from build123d import *

# Parameters (mm, degrees)
BOSS_EXTRUDE1_DEPTH     = 16.316743
CUT_EXTRUDE1_DEPTH      = 16.04
CUT_EXTRUDE1_DEPTH_BACK = 16.96
CUT_EXTRUDE2_DEPTH      = 29
CUT_EXTRUDE2_DEPTH_BACK = 29


with BuildPart() as part:
    # Sketch3 → Boss-Extrude1 (new body)
    with BuildSketch(Plane(origin=(0, 0, 0), x_dir=(1, 0, 0), z_dir=(0, 1, 0))):
        Polygon((-28, 15.96), (28, 15.96), (28, -15.04), (12.57, -15.04), (8.79, -11.59), (8.79, -11.02), (12.24, -7.24), (12.24, 0), (-12.24, 0), (-12.24, -7.24), (-8.79, -11.02), (-8.79, -11.59), (-12.57, -15.04), (-28, -15.04), align=None)
    extrude(amount=-BOSS_EXTRUDE1_DEPTH)

    # Sketch4 → Cut-Extrude1 (cut, two sides)
    with BuildSketch(Plane.XY) as cut_extrude1_sk:
        Polygon((28, -3.175), (28, -4.282415891), (20.400144244, -3.728707945), align=None)
        Polygon((28, -4.282415891), (28, -5.389831781), (20.400144244, -4.836123836), align=None)
        Polygon((28, -5.389831781), (28, -6.497247672), (20.400144244, -5.943539726), align=None)
        Polygon((28, -6.497247672), (28, -7.604663562), (20.400144244, -7.050955617), align=None)
        Polygon((28, -7.604663562), (28, -8.712079453), (20.400144244, -8.158371507), align=None)
        Polygon((28, -8.712079453), (28, -9.819495343), (20.400144244, -9.265787398), align=None)
        Polygon((20.400144244, -10.373203288), (28, -10.926911234), (28, -9.819495343), align=None)
        Polygon((28, -10.926911234), (28, -12.034327124), (20.400144244, -11.480619179), align=None)
        Polygon((28, -12.034327124), (28, -13.141743015), (20.400144244, -12.588035069), align=None)
        Polygon((-28, -13.141743015), (-28, -12.034327124), (-20.400144244, -12.588035069), align=None)
        Polygon((-28, -10.926911234), (-20.400144244, -11.480619179), (-28, -12.034327124), align=None)
        Polygon((-28, -10.926911234), (-28, -9.819495343), (-20.400144244, -10.373203288), align=None)
        Polygon((-28, -8.712079453), (-20.400144244, -9.265787398), (-28, -9.819495343), align=None)
        Polygon((-28, -7.604663562), (-20.400144244, -8.158371507), (-28, -8.712079453), align=None)
        Polygon((-28, -6.497247672), (-20.400144244, -7.050955617), (-28, -7.604663562), align=None)
        Polygon((-28, -5.389831781), (-20.400144244, -5.943539726), (-28, -6.497247672), align=None)
        Polygon((-28, -4.282415891), (-20.400144244, -4.836123836), (-28, -5.389831781), align=None)
        Polygon((-28, -3.175), (-20.400144244, -3.728707945), (-28, -4.282415891), align=None)
    extrude(amount=CUT_EXTRUDE1_DEPTH, mode=Mode.SUBTRACT)
    extrude(cut_extrude1_sk.sketch, amount=-CUT_EXTRUDE1_DEPTH_BACK, mode=Mode.SUBTRACT)

    # Sketch5 → Cut-Extrude2 (cut, two sides)
    with BuildSketch(Plane(origin=(0, 0, 0), x_dir=(0, 0, -1), z_dir=(1, 0, 0))) as cut_extrude2_sk:
        Polygon((15.96, -3.175), (15.96, -4.282415891), (8.360144244, -3.728707945), align=None)
        Polygon((8.360144244, -4.836123836), (15.96, -5.389831781), (15.96, -4.282415891), align=None)
        Polygon((15.96, -5.389831781), (15.96, -6.497247672), (8.360144244, -5.943539726), align=None)
        Polygon((8.360144244, -7.050955617), (15.96, -7.604663562), (15.96, -6.497247672), align=None)
        Polygon((15.96, -7.604663562), (15.96, -8.712079453), (8.360144244, -8.158371507), align=None)
        Polygon((8.360144244, -9.265787398), (15.96, -9.819495343), (15.96, -8.712079453), align=None)
        Polygon((15.96, -9.819495343), (15.96, -10.926911234), (8.360144244, -10.373203288), align=None)
        Polygon((8.360144244, -11.480619179), (15.96, -12.034327124), (15.96, -10.926911234), align=None)
        Polygon((15.96, -12.034327124), (15.96, -13.141743015), (8.360144244, -12.588035069), align=None)
    extrude(amount=CUT_EXTRUDE2_DEPTH, mode=Mode.SUBTRACT)
    extrude(cut_extrude2_sk.sketch, amount=-CUT_EXTRUDE2_DEPTH_BACK, mode=Mode.SUBTRACT)


solid = part.part
Part model, mm, in its own coordinate system. Give positions to 0.01 mm unless a question says otherwise; leave off trailing zeros. Loops run counter-clockwise (first coordinate to the right, second up) from the corner with the lowest first, then second, coordinate; pieces in that order, holes last.
(1) Band-saw the part on D-D (x = 17.5). Write the cut outline in (y, z) (1 decimal).
Return value:
outline: (-16.3, -16) - (-13.1, -16) - (-12.6, -8.4) - (-12, -16) - (-11.5, -8.4) - (-10.9, -16) - (-10.4, -8.4) - (-9.8, -16) - (-9.3, -8.4) - (-8.7, -16) - (-8.2, -8.4) - (-7.6, -16) - (-7.1, -8.4) - (-6.5, -16) - (-5.9, -8.4) - (-5.4, -16) - (-4.8, -8.4) - (-4.3, -16) - (-3.7, -8.4) - (-3.2, -16) - (0, -16) - (0, 15) - (-16.3, 15) - close
(2) Pin check, flat tips, straight feed: pin 1 (6 mm diameter, centred on y = -8.5, z = 3, fed in from -X); pin 2 (6 mm diameter, centred on y = -8.5, z = 4.5, fed in from +X). Stop position of each tip, or through.
Return value:
pin 1: stops at x = -28
pin 2: stops at x = 28
(3) Band-saw the part on A-A (x = 11). Write the cut outline in (y, z) (1 decimal), and give its area (3 significant figures).
Return value:
outline: (-16.3, -16) - (-13.1, -16) - (-12.6, -8.4) - (-12, -16) - (-11.5, -8.4) - (-10.9, -16) - (-10.4, -8.4) - (-9.8, -16) - (-9.3, -8.4) - (-8.7, -16) - (-8.2, -8.4) - (-7.6, -16) - (-7.1, -8.4) - (-6.5, -16) - (-5.9, -8.4) - (-5.4, -16) - (-4.8, -8.4) - (-4.3, -16) - (-3.7, -8.4) - (-3.2, -16) - (0, -16) - (0, 0) - (-16.3, 0) - close; (-16.3, 8.6) - (0, 8.6) - (0, 13.6) - (-16.3, 13.6) - close
area: 304 mm2
(4) Band-saw the part on B-B (x = 2). Write the cut outline in (y, z) (1 decimal).
Return value:
outline: (-16.3, -16) - (-13.1, -16) - (-12.6, -8.4) - (-12, -16) - (-11.5, -8.4) - (-10.9, -16) - (-10.4, -8.4) - (-9.8, -16) - (-9.3, -8.4) - (-8.7, -16) - (-8.2, -8.4) - (-7.6, -16) - (-7.1, -8.4) - (-6.5, -16) - (-5.9, -8.4) - (-5.4, -16) - (-4.8, -8.4) - (-4.3, -16) - (-3.7, -8.4) - (-3.2, -16) - (0, -16) - (0, 0) - (-16.3, 0) - close
(5) Drill centre lines: line 1 along Z through (x, y) = (-10, -2.5); line 2 along Z through (x, y) = (5.5, -15.5); line 3 along X through (y, z) = (-1.5, 13.5). Where is each one in solid material? Low to high.
Return value:
line 1: z = -15.96 to 0, 9.69 to 12.69
line 2: z = -15.96 to 0
line 3: x = -28 to -10.88, 10.88 to 28
(6) Pull direction Y, two halves, no side cores. Call faces 1 (the flat face through (0, -15, -15.96)), 2 (the flat face through (-24.25, -11.2, 3.2)): pulls with the +Y half, pulls with the -Y half, needs draft (parallel to the pull), parting line crosses it, or undercut.
Return value:
face 1: needs draft
face 2: undercut
(7) Band-saw the part on C-C (z = -10.5). Count the separate pieces of the cut face and the enclosed holes in it, and give its area (3 significant figures).
Return value:
separate pieces: 10
enclosed holes: 0
area: 717 mm2
